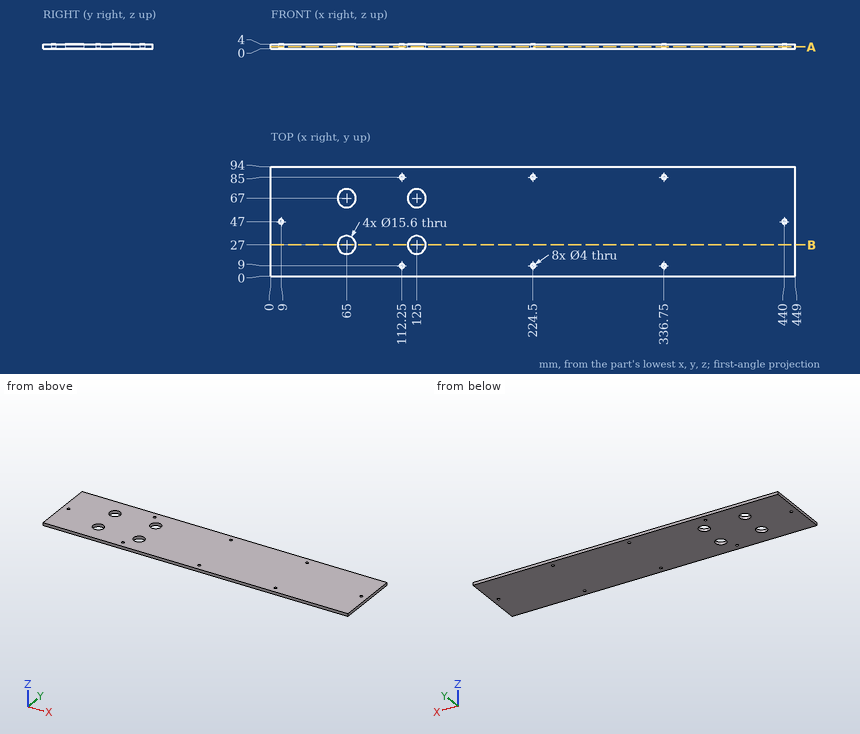
Can you work these out from the drawing? Everything is in mm from the part's minimum corner. Round coordinates to 2 decimals unless told otherwise and drop trailing zeros. Write each loop counter-clockwise with the first axis right and the second up, starting at its lowest first coordinate (ties: lowest second). Pieces come first, ordered by that corner, then holes. Notation, with made-up numbers: (-15.5, -14) - (36.5, -14) arc R17 cw to (36.5, 7) - close; hole circle Ø11 at (61, 31.25). An arc over 180 degrees is marked (long way). Use a Markdown table: item, result.
Q1. For pin 1 (3 mm diameter, centred on x = 224.5, y = 9, fed in from -Z), with a flat end and sliding along its axis, tell me the tip position at first contact or that it passes through.
Output values:
| item | result |
|---|---|
| pin 1 | through |
Q2. I want a section at B-B (y = 27). List the corners of the cut face in (x, z) for me, plus the area to 3 significant figures.
Output values:
| item | result |
|---|---|
| outline | (0, 0) - (57.2, 0) - (57.2, 4) - (0, 4) - close; (72.8, 0) - (117.2, 0) - (117.2, 4) - (72.8, 4) - close; (132.8, 0) - (449, 0) - (449, 4) - (132.8, 4) - close |
| area | 1,670 mm2 |
Q3. Please list where these lines run through material, in increasing order: L1, parallel to X at y = 26, z = 1.55; L2, parallel to Y at x = 336.75, z = 1.8; L3, parallel to Y at x = 125, z = 3.1.
Output values:
| item | result |
|---|---|
| L1 | 0 to 57.26, 72.74 to 117.26, 132.74 to 449 |
| L2 | 0 to 7, 11 to 83, 87 to 94 |
| L3 | 0 to 19.2, 34.8 to 59.2, 74.8 to 94 |
Q4. I want a section at A-A (z = 1.45). Count the separate pieces of the cut face and the enclosed holes in it, plus the area to 3 significant figures.
Output values:
| item | result |
|---|---|
| separate pieces | 1 |
| enclosed holes | 12 |
| area | 41,300 mm2 |
